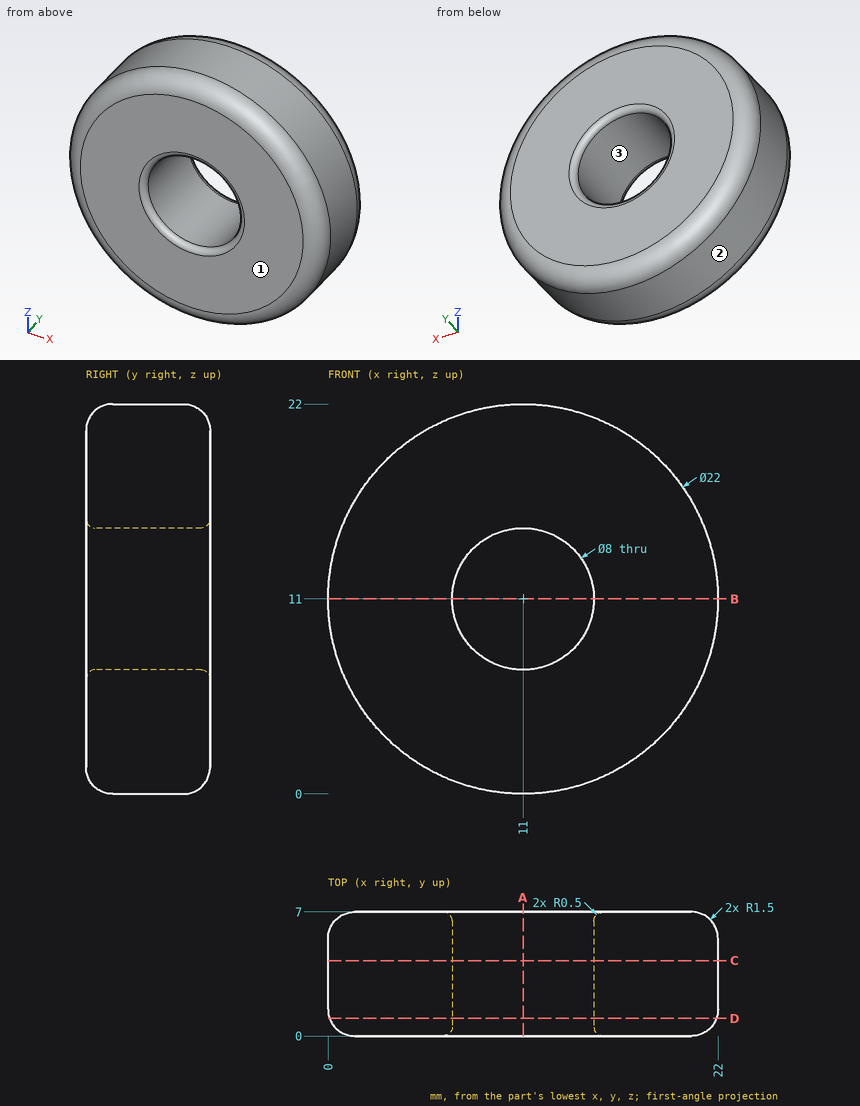
The drawing under review shows one solid part. Ordinate dimensions are in mm from its lowest x, y, z. Coordinates: 2 decimals unless noted, no trailing zeros. Order: outer loops, then holes, each group sorted by start corner. A loop starts at its lowest first (then second) coordinate and runs counter-clockwise, first axis right, second up. Notation, with made-up numbers: (-38.75, 9) -> (6.25, 9) arc R11 cw to (6.25, 29) -> close; hole circle Ø8 at (43, 14.25). An arc over 180 degrees is marked (long way). Answer in a Markdown table with one row per item. Add a question column.
Item 1: We need section A-A on x = 11. Write out the cut boundary in (y, z).
Item 2: Clearance check with flat-ended pins moving along their axes: pin 1 (3 mm diameter, centred on x = 5.5, y = 4, fed in from +Z); pin 2 (1.5 mm diameter, centred on x = 9.5, y = 5, fed in from -Z); pin 3 (5 mm diameter, centred on x = 11, z = 11, fed in from -Y). State where each tip first meets the part, or that it passes through.
Item 3: We need section D-D on y = 1. Write out the cut boundary in (x, z).
Item 4: We need section C-C on y = 4.25. Write out the cut boundary in (x, z), plus the area to 3 significant figures.
Item 5: Mouldability with a two-part tool opening along X and no side actions: class the marked faces 1, 2 and 3 as +X half, -X half, draft (parallel to the pull), parting line (faces both ways), or undercut.
Item 6: We need section B-B on z = 11. Write out the cut boundary in (x, y).
Item 7: To check wall thickness, follow probe 1 along X at (y, z) = (2.15, 11); probe 2 along X at (y, z) = (1.5, 8); probe 3 along Z at (x, y) = (9, 6.5). State the ranges of each line that lie inside material, in increasing order.
Final values:
| question | item | result |
|---|---|---|
| 1 | outline | (0, 1.5) arc R1.5 ccw to (1.5, 0) -> (5.5, 0) arc R1.5 ccw to (7, 1.5) -> (7, 6.5) arc R0.5 ccw to (6.5, 7) -> (0.5, 7) arc R0.5 ccw to (0, 6.5) -> close; (0, 15.5) arc R0.5 ccw to (0.5, 15) -> (6.5, 15) arc R0.5 ccw to (7, 15.5) -> (7, 20.5) arc R1.5 ccw to (5.5, 22) -> (1.5, 22) arc R1.5 ccw to (0, 20.5) -> close |
| 2 | pin 1 | stops at z = 21.25 |
| 2 | pin 2 | stops at z = 0.03 |
| 2 | pin 3 | passes through |
| 3 | outline | circle Ø21.83 at (11, 11); hole circle Ø8 at (11, 11) |
| 4 | outline | circle Ø22 at (11, 11); hole circle Ø8 at (11, 11) |
| 4 | area | 330 mm2 |
| 5 | face 1 | draft |
| 5 | face 2 | parting line |
| 5 | face 3 | undercut |
| 6 | outline | (0, 1.5) arc R1.5 ccw to (1.5, 0) -> (6.5, 0) arc R0.5 ccw to (7, 0.5) -> (7, 6.5) arc R0.5 ccw to (6.5, 7) -> (1.5, 7) arc R1.5 ccw to (0, 5.5) -> close; (15, 0.5) arc R0.5 ccw to (15.5, 0) -> (20.5, 0) arc R1.5 ccw to (22, 1.5) -> (22, 5.5) arc R1.5 ccw to (20.5, 7) -> (15.5, 7) arc R0.5 ccw to (15, 6.5) -> close |
| 7 | probe 1 | x = 0 to 7, 15 to 22 |
| 7 | probe 2 | x = 0.42 to 8.35, 13.65 to 21.58 |
| 7 | probe 3 | z = 0.57 to 7.54, 14.46 to 21.43 |
